from build123d import *

# Parameters (mm, degrees)
F1_DEPTH = 100
F2_W     = 20
F2_H     = 89.4427191
F3_DEPTH = 10
F4_DEPTH = 10
F5_DEPTH = 10
F6_DEPTH = 10


with BuildPart() as f1:
    # F0 (on Front) → F1 (new body)
    with BuildSketch(Plane.XZ):
        Polygon((0, 100), (0, 0), (100, 0), (100, 20), (60, 100), (40, 100), (40, 80), (20, 80), (20, 100), align=None)
    extrude(amount=F1_DEPTH)

    # F2 (on face) → F3 (cut)
    with BuildSketch(Plane(origin=(88, 0, 44), x_dir=(0, 1, 0), z_dir=(0.894427191, 0, 0.4472135955))):
        with Locations((-50, 17.88854382)):
            Rectangle(F2_W, F2_H)
    extrude(amount=-F3_DEPTH, mode=Mode.SUBTRACT)

    # F4 (cut): a face of the model
    f4_faces = [f1.faces().sort_by_distance(p)[0] for p in [
        (55.527864045, -50, 97.7639320225),
    ]]
    extrude(f4_faces, amount=-F4_DEPTH, mode=Mode.SUBTRACT)

    # F5 (cut): a face of the model
    f5_faces = [f1.faces().sort_by_distance(p)[0] for p in [
        (95.527864045, -50, 17.7639320225),
    ]]
    extrude(f5_faces, amount=-F5_DEPTH, mode=Mode.SUBTRACT)

    # F6 (cut): a face of the model
    f6_faces = [f1.faces().sort_by_distance(p)[0] for p in [
        (97.7639320225, -50, 7.7016261238),
    ]]
    extrude(f6_faces, amount=-F6_DEPTH, mode=Mode.SUBTRACT)


solid = f1.part
Build history of the part. All positions in model axes, mm. A direction names the side the tool comes from. Give positions to 0.01 mm unless a question says otherwise; leave off trailing zeros. Loops run counter-clockwise (first coordinate to the right, second up) from the corner with the lowest first, then second, coordinate; pieces in that order, holes last. Notation, with made-up numbers: (-9.5, 87.25) -> (18.5, 87.25) arc R19 cw to (18.5, 97.25) -> close; hole circle Ø11 at (-12.5, 78). An arc over 180 degrees is marked (long way). Answer in a Markdown table with one row per item.
Item 1: Slice it at C-C on x = 91.5. Write the cut outline in (y, z), plus the area to 3 significant figures.
Findings below:
| item | result |
|---|---|
| outline | (-100, 0) -> (0, 0) -> (0, 37) -> (-40, 37) -> (-40, 14.64) -> (-60, 14.64) -> (-60, 37) -> (-100, 37) -> close |
| area | 3,250 mm² |
Item 2: Slice it at B-B on z = 16. Write the cut outline in (x, y).
Findings below:
| item | result |
|---|---|
| outline | (0, -100) -> (100, -100) -> (100, -60) -> (90.82, -60) -> (90.82, -40) -> (100, -40) -> (100, 0) -> (0, 0) -> close |
Item 3: Tool access for faces 5 (the flat face through (40, -49, 90)), 6 (the flat face through (78, -60, 53)), 7 (the flat face through (10, -49, 100)): list every direction of +Z, -Z, +X, -X, +Y, -Y with a clear straight run to the whole face (end or side of a thin tool).
Findings below:
| item | result |
|---|---|
| face 5 | +Z, +Y, -Y |
| face 6 | +Z, +X |
| face 7 | +Z, +X, -X, +Y, -Y |
Item 4: Flat gauge pins, fed straight in: P1, Ø16, axis at x = 31, y = -44.5, coming from the +Z side; P2, Ø1.5, axis at y = -36, z = 75, coming from the +X side (3 decimals); P3, Ø16, axis at y = -34.5, z = 93.5, coming from the +X side. Where does each tip first touch, or does it go through?
Findings below:
| item | result |
|---|---|
| P1 | stops at z = 80 |
| P2 | stops at x = 72.875 |
| P3 | stops at x = 67.25 |
Item 5: Slice it at A-A on y = -66.5. Write the cut outline in (x, z), plus the area to 3 significant figures.
Findings below:
| item | result |
|---|---|
| outline | (0, 0) -> (100, 0) -> (100, 20) -> (60, 100) -> (40, 100) -> (40, 80) -> (20, 80) -> (20, 100) -> (0, 100) -> close |
| area | 8,000 mm² |
Item 6: Mould opens along Y. For faces 1 (the flat face through (38, -100, 40)), 2 (the flat face through (48, -49, 100)), 3 (the flat face through (78, -40, 53)), 4 (the flat face through (73.47, -50.14, 50.7)) say: pulls with the +Y half, pulls with the -Y half, needs draft (parallel to the pull), parting line crosses it, or undercut.
Findings below:
| item | result |
|---|---|
| face 1 | pulls with the -Y half |
| face 2 | needs draft |
| face 3 | undercut |
| face 4 | undercut |
Item 7: Probe line 1 along Z through (x, y) = (38, -35.5); line 2 along X through (y, z) = (-51.5, 83.5); line 3 along X through (y, z) = (-84, 81). List the from-to ranges inside material, lowest first. Write a range as [from, to].
Findings below:
| item | result |
|---|---|
| line 1 | z = [0, 80] |
| line 2 | x = [0, 20], [40, 57.07] |
| line 3 | x = [0, 20], [40, 69.5] |
Item 8: Slice it at D-D on x = 33. Write the cut outline in (y, z), plus the area to 3 significant figures.
Findings below:
| item | result |
|---|---|
| outline | (-100, 0) -> (0, 0) -> (0, 80) -> (-100, 80) -> close |
| area | 8,000 mm² |
